Here's how the part is built. I have some questions about the finished solid (model axes, mm). A direction names the side the tool comes from. Round coordinates to 2 decimals unless told otherwise and drop trailing zeros. Loops run counter-clockwise (first coordinate to the right, second up) from the corner with the lowest first, then second, coordinate; pieces in that order, holes last. Notation, with made-up numbers: M 89,6 L 93,6 A12 cw 93,20 Z; hole C 38,13.25 d2. An arc over 180 degrees is marked long. Answer as a JSON object with one key per item and string values.
from build123d import *

# Parameters (mm, degrees)
SKETCH1_R           = 32.750000032
BOSS_EXTRUDE1_DEPTH = 26.199999924
SKETCH3_R           = 22.749999966
CUT_EXTRUDE1_DEPTH  = 8.399999964
CUT_EXTRUDE2_DEPTH  = 4.49999989


with BuildPart() as part:
    # Sketch1 → Boss-Extrude1 (new body)
    with BuildSketch(Plane(origin=(0, 0, 0), x_dir=(1, 0, 0), z_dir=(0, 1, 0))):
        with Locations(Location((0, 0, 0), (0, 0, 270))):
            Circle(SKETCH1_R)
    extrude(amount=BOSS_EXTRUDE1_DEPTH)

    # Sketch3 → Cut-Extrude1 (cut)
    with BuildSketch(Plane.XZ):
        with Locations(Location((0, 0, 0), (0, 0, 270))):
            Circle(SKETCH3_R)
    extrude(amount=-CUT_EXTRUDE1_DEPTH, mode=Mode.SUBTRACT)

    # Sketch4 → Cut-Extrude2 (cut)
    with BuildSketch(Plane.XZ.offset(-8.399999964)):
        Polygon((-5.851405972, -3.709588544), (0.286894931, -6.922260491), (6.138300902, -3.212671947), (5.851405972, 3.709588544), (-0.286894931, 6.922260491), (-6.138300902, 3.212671947), align=None)
    extrude(amount=-CUT_EXTRUDE2_DEPTH, mode=Mode.SUBTRACT)


solid = part.part
Item 1: I want a section at D-D on y = 23.5. List the corners of the cut face in (x, z) for me, plus the area to 3 significant figures.
Solution:
{"outline": "C 0,0 d65.5", "area": "3,370 mm2"}
Item 2: If I drill on L1, parallel to X at y = 5.75, z = 0; L2, parallel to Y at x = 3, z = -7; L3, parallel to X at y = 2.25, z = -8, over which ranges is the centre line in solid material (lowest first)? Write a range as from..to.
Solution:
{"L1": "x = -32.75..-22.75, 22.75..32.75", "L2": "y = 8.4..26.2", "L3": "x = -31.76..-21.3, 21.3..31.76"}
Item 3: I want a section at B-B on x = 10.5. List the corners of the cut face in (y, z) for me, plus the area to 3 significant figures.
Solution:
{"outline": "M 0,-31.02 L 26.2,-31.02 L 26.2,31.02 L 0,31.02 L 0,20.18 L 8.4,20.18 L 8.4,-20.18 L 0,-20.18 Z", "area": "1,290 mm2"}
Item 4: We'd pull the mould along X, two halves only. Please class faces 3 (the face through (0, 26.2, 0)), 4 (the face through (5.997, 10.618, 0.2)), 5 (the face through (1.44, 12.92, -32.72)): +X half, -X half, draft (parallel to the pull), parting line (faces both ways), or undercut.
Solution:
{"face 3": "draft", "face 4": "undercut", "face 5": "parting line"}
Item 5: For faces 1 (the face through (2.83, 10.62, 5.29)), 2 (the face through (-7, 0, -22)), which set-ups out of +Z, -Z, +X, -X, +Y, -Y let a thin tool reach every point of the face, with its end or its side?
Solution:
{"face 1": "-Y", "face 2": "+Z, -Z, +X, -X, -Y"}
Item 6: I want a section at C-C on z = -21.5. List the corners of the cut face in (x, y) for me.
Solution:
{"outline": "M -24.7,0 L -7.44,0 L -7.44,8.4 L 7.44,8.4 L 7.44,0 L 24.7,0 L 24.7,26.2 L -24.7,26.2 Z"}
Item 7: I want a section at A-A on y = 11. List the corners of the cut face in (x, z) for me, plus the area to 3 significant figures.
Solution:
{"outline": "C 0,0 d65.5; hole M -6.14,3.21 L -5.85,-3.71 L 0.29,-6.92 L 6.14,-3.21 L 5.85,3.71 L -0.29,6.92 Z", "area": "3,240 mm2"}
Item 8: For P1, Ø13.5, axis at x = -1, z = -0.5, coming from the -Y side; P2, Ø10, axis at x = 15, y = 22.5, coming from the -Z side; P3, Ø12, axis at x = -25, y = 15, coming from the -Z side, each with a flat end and sliding along its axis, tell me the tip position at first contact or that it passes through.
Solution:
{"P1": "stops at y = 8.4", "P2": "stops at z = -31.19", "P3": "stops at z = -26.68"}
